The figure shows three views and two pictorial views of one solid part (mm, origin at its lowest corner). Answer the questions. Round coordinates to 2 decimals unless told otherwise and drop trailing zeros. Loops run counter-clockwise (first coordinate to the right, second up) from the corner with the lowest first, then second, coordinate; pieces in that order, holes last. Notation, with made-up numbers: (-24.75, 18.5) -> (7.25, 18.5) arc R31 ccw to (7.25, 56.5) -> close; hole circle Ø3 at (-10.5, 53). An arc over 180 degrees is marked (long way). Use a Markdown table: item, result. Add a question column.
Q1. Section A-A on x = 26.5 is taken. Give the vertices of the cut face in (y, z) (1 decimal).
Q2. Consider line 1 (Z direction, x = 44, y = 0.25) (3 decimals); line 2 (X direction, y = 0.35, z = 42); line 3 (X direction, y = 0.25, z = 52.5) (3 decimals). Determine where each line is inside the solid, lowest interval first.
Q3. Section B-B on z = 33.5 is taken. Give the vertices of the cut face in (x, y) (1 decimal).
Q4. Given pin 1 Ø1 at (x, y) = (1.5, 1.5) entering from +Z (3 decimals); pin 2 Ø1.6 at (x, y) = (2, 2) entering from -Z (3 decimals); pin 3 Ø1 at (y, z) = (1.5, 22) entering from +X, each flat-ended and moving along its own axis, determine where each tip first touches the part or whether it passes through.
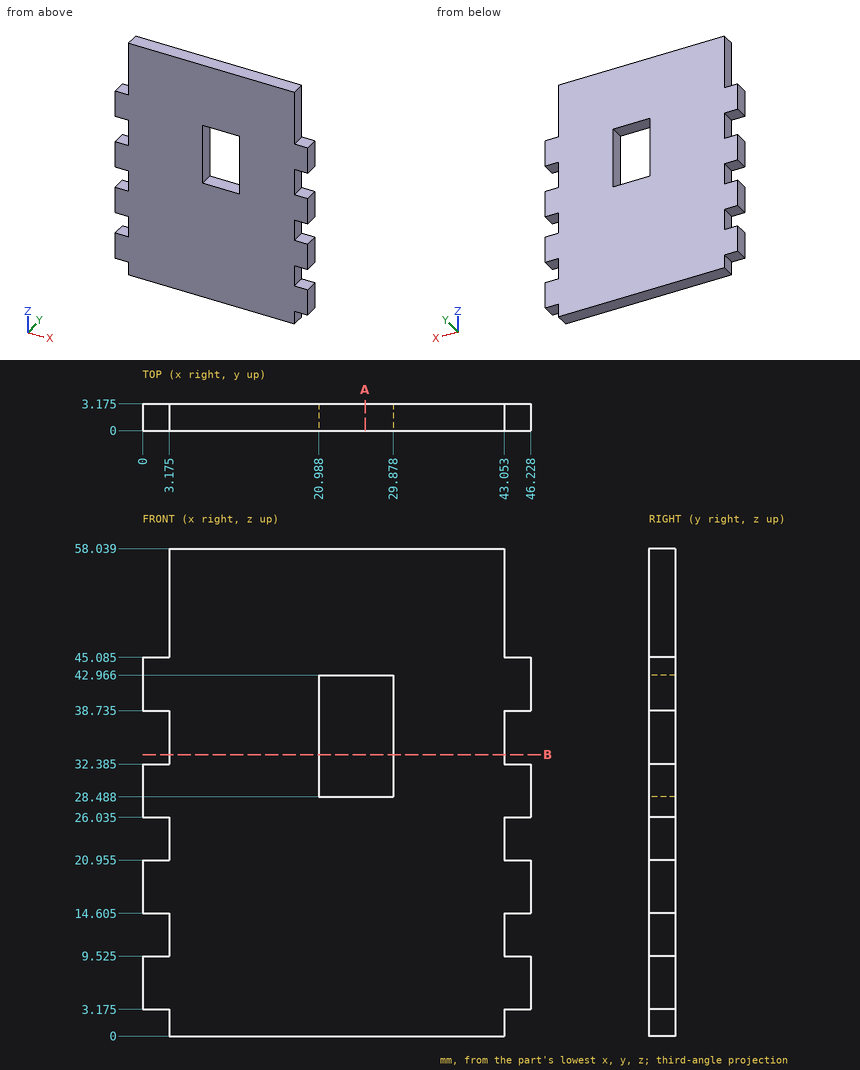
Checked values:
| question | item | result |
|---|---|---|
| 1 | outline | (0, 0) -> (3.2, 0) -> (3.2, 28.5) -> (0, 28.5) -> close; (0, 43) -> (3.2, 43) -> (3.2, 58) -> (0, 58) -> close |
| 2 | line 1 | z = 3.175 to 9.525, 14.605 to 20.955, 26.035 to 32.385, 38.735 to 45.085 |
| 2 | line 2 | x = 0 to 20.99, 29.88 to 46.23 |
| 2 | line 3 | x = 3.175 to 43.053 |
| 3 | outline | (3.2, 0) -> (21, 0) -> (21, 3.2) -> (3.2, 3.2) -> close; (29.9, 0) -> (43.1, 0) -> (43.1, 3.2) -> (29.9, 3.2) -> close |
| 4 | pin 1 | stops at z = 45.085 |
| 4 | pin 2 | stops at z = 3.175 |
| 4 | pin 3 | stops at x = 43.05 |
